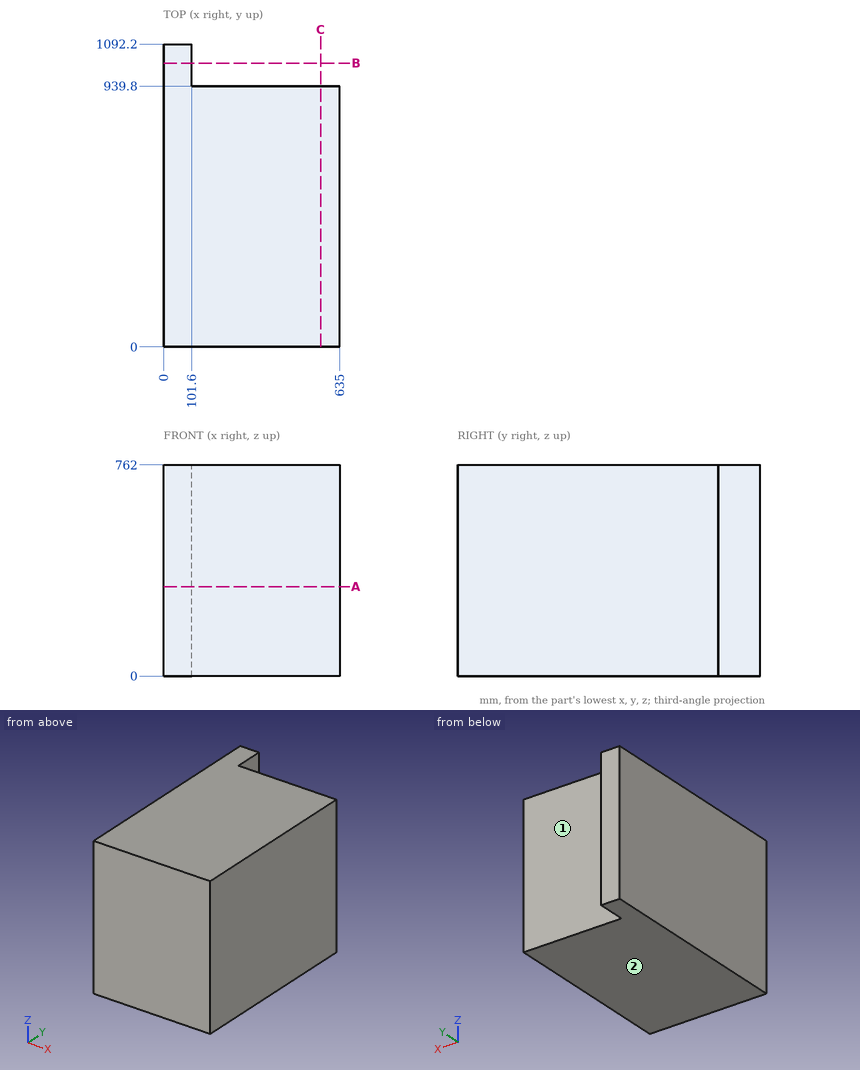
Source: three-view drawing plus pictorial views. Frame: mm from the lowest corner of the part. A direction names the side the tool comes from. Round coordinates to 2 decimals unless told otherwise and drop trailing zeros. Loops run counter-clockwise (first coordinate to the right, second up) from the corner with the lowest first, then second, coordinate; pieces in that order, holes last.
1. Section query A-A on z = 322. Output: boundary loops of the cut face in (x, y).
2. Section query C-C on x = 566. Output: boundary loops of the cut face in (y, z).
3. Section query B-B on y = 1023. Output: boundary loops of the cut face in (x, z).
4. Ray query, L1, parallel to Y at x = 481, z = 228.5. Return the intervals inside material, ascending.
5. Access query for the marked faces 1 and 2. Directions: +Z, -Z, +X, -X, +Y, -Y. A direction counts if a zero-diameter tool reaches every point of the face in a straight line with its end or side. Return the directions, or none.
Answers below:
1. outline: (0, 0) - (635, 0) - (635, 939.8) - (101.6, 939.8) - (101.6, 1092.2) - (0, 1092.2) - close
2. outline: (0, 0) - (939.8, 0) - (939.8, 762) - (0, 762) - close
3. outline: (0, 0) - (101.6, 0) - (101.6, 762) - (0, 762) - close
4. L1: y = 0 to 939.8
5. face 1: +Z, -Z, +X, +Y
5. face 2: -Z, +X, -X, +Y, -Y
